```python
from build123d import *

# Parameters (mm, degrees)
SKETCH1_W           = 252.4
SKETCH1_H           = 125
BOSS_EXTRUDE1_DEPTH = 23.5
SKETCH2_W           = 227
SKETCH2_H           = 102
CUT_EXTRUDE1_DEPTH  = 5
SKETCH3_W           = 227
SKETCH3_H           = 85
CUT_EXTRUDE2_DEPTH  = 7
SKETCH4_W           = 12.7
SKETCH4_H           = 85
CUT_EXTRUDE3_DEPTH  = 12
SKETCH5_W           = 12.7
SKETCH5_H           = 85
CUT_EXTRUDE4_DEPTH  = 12
FILLET1_R           = 1


with BuildPart() as part:
    # Sketch1 → Boss-Extrude1 (new body)
    with BuildSketch(Plane(origin=(0, 0, 0), x_dir=(1, 0, 0), z_dir=(0, 1, 0))):
        with Locations((126.2, 62.5)):
            Rectangle(SKETCH1_W, SKETCH1_H)
    extrude(amount=BOSS_EXTRUDE1_DEPTH)

    # Sketch2 → Cut-Extrude1 (cut)
    with BuildSketch(Plane(origin=(0, 23.5, 0), x_dir=(1, 0, 0), z_dir=(0, 1, 0))):
        with Locations((126.2, 63.7)):
            Rectangle(SKETCH2_W, SKETCH2_H)
    extrude(amount=-CUT_EXTRUDE1_DEPTH, mode=Mode.SUBTRACT)

    # Sketch3 → Cut-Extrude2 (cut)
    with BuildSketch(Plane(origin=(0, 18.5, 0), x_dir=(1, 0, 0), z_dir=(0, 1, 0))):
        with Locations((126.2, 63.65)):
            Rectangle(SKETCH3_W, SKETCH3_H)
    extrude(amount=-CUT_EXTRUDE2_DEPTH, mode=Mode.SUBTRACT)

    # Sketch4 → Cut-Extrude3 (cut)
    with BuildSketch(Plane(origin=(0, 23.5, 0), x_dir=(1, 0, 0), z_dir=(0, 1, 0))):
        with Locations((6.35, 63.65)):
            Rectangle(SKETCH4_W, SKETCH4_H)
    extrude(amount=-CUT_EXTRUDE3_DEPTH, mode=Mode.SUBTRACT)

    # Sketch5 → Cut-Extrude4 (cut)
    with BuildSketch(Plane(origin=(0, 23.5, 0), x_dir=(1, 0, 0), z_dir=(0, 1, 0))):
        with Locations((246.05, 63.65)):
            Rectangle(SKETCH5_W, SKETCH5_H)
    extrude(amount=-CUT_EXTRUDE4_DEPTH, mode=Mode.SUBTRACT)

    # Fillet1
    fillet1_edges = [part.edges().sort_by_distance(p)[0] for p in [
        (12.7, 18.5, -110.425),
        (12.7, 21, -12.7),
        (126.2, 18.5, -114.7),
        (12.7, 21, -114.7),
        (239.7, 18.5, -16.925),
        (239.7, 21, -114.7),
        (126.2, 18.5, -12.7),
        (239.7, 21, -12.7),
        (12.7, 18.5, -16.925),
        (239.7, 18.5, -110.425),
        (126.2, 11.5, -21.15),
        (126.2, 11.5, -106.15),
    ]]
    fillet(fillet1_edges, radius=FILLET1_R)


solid = part.part
```
Check sheet for the modelled part. Datum: model origin and axes. Units: mm. A direction names the side the tool comes from. Give positions to 0.01 mm unless a question says otherwise; leave off trailing zeros. Write each loop counter-clockwise with the first axis right and the second up, starting at its lowest first coordinate (ties: lowest second). Pieces come first, ordered by that corner, then holes.
Item 1: Access from +Z, -Z, +X, -X, +Y, -Y to the whole of each face (thin tool, end or side, straight path). Record for faces 1 (the face through (124, 11.5, -64)), 2 (the face through (125, 18.5, -110)), 3 (the face through (124, 12, -125)).
Item 2: Draft check along X on faces 4 (the face through (125, 18.5, -17)), 5 (the face through (0, 9, -62)), 6 (the face through (124, 16, -21.15)). Enter one of: released by +X, released by -X, zero draft, split by the parting line, or undercut.
Item 3: Cross-section at B-B (z = -84). Enter the section's corners in (x, y), and give its area (3 significant figures).
Item 4: Gauge pin test, flat ends, axial feed: pin 1 (10 mm diameter, centred on y = 19.5, z = -91.5, fed in from +X); pin 2 (3.5 mm diameter, centred on x = 78, z = -18.5, fed in from +Y). Record the tip position at first contact, or that the pin passes through.
Item 5: Scan lines: L1, parallel to Z at x = 126, y = 22; L2, parallel to Z at x = 223.5, y = 17.75; L3, parallel to Y at x = 107.5, z = -29.5. Record each from-to range of solid material in increasing order.
Item 6: Cross-section at A-A (x = 157). Enter the section's corners in (y, z).
Report:
1. face 1: +X, -X, +Y
1. face 2: +Y
1. face 3: -Z, +X, -X, +Y, -Y
2. face 4: undercut
2. face 5: released by -X
2. face 6: zero draft
3. outline: (0, 0) - (252.4, 0) - (252.4, 11.5) - (0, 11.5) - close
3. area: 2,900 mm2
4. pin 1: passes through
4. pin 2: stops at y = 18.5
5. L1: z = -125 to -114.7, -12.7 to 0
5. L2: z = -125 to -106.15, -21.15 to 0
5. L3: y = 0 to 11.5
6. outline: (0, -125) - (23.5, -125) - (23.5, -114.7) - (19.5, -114.7) arc R1 cw to (18.5, -113.7) - (18.5, -106.15) - (12.5, -106.15) arc R1 cw to (11.5, -105.15) - (11.5, -22.15) arc R1 cw to (12.5, -21.15) - (18.5, -21.15) - (18.5, -13.7) arc R1 cw to (19.5, -12.7) - (23.5, -12.7) - (23.5, 0) - (0, 0) - close
